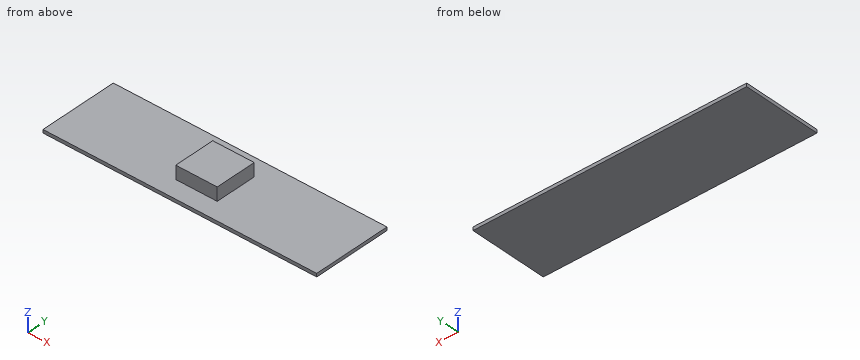
Autodesk Fusion 360 part; units mm, degrees
sketch "Sketch1" plane through (0, 0, 0) normal (0, 0, 1) x (1, 0, 0)
  line L0 (16.5, -4.75) -> (-16.5, -4.75)
  line L1 (-16.5, -4.75) -> (-16.5, 4.75)
  line L2 (-16.5, 4.75) -> (16.5, 4.75)
  line L3 (16.5, 4.75) -> (16.5, -4.75)
  line L4 (16.5, -4.75) -> (-16.5, 4.75) construction
  line L5 (-16.5, -4.75) -> (16.5, 4.75) construction
  line L6 (2.5, -2.5) -> (-2.5, -2.5)
  line L7 (-2.5, -2.5) -> (-2.5, 2.5)
  line L8 (-2.5, 2.5) -> (2.5, 2.5)
  line L9 (2.5, 2.5) -> (2.5, -2.5)
  line L10 (2.5, -2.5) -> (-2.5, 2.5) construction
  line L11 (-2.5, -2.5) -> (2.5, 2.5) construction
  dimension "d1" = 14
  dimension "d2" = 14
  dimension "d3" = 5
  dimension "d4" = 5
  dimension "d5" = 9.5
  dimension "d6" = 33
extrude "Extrude1" add sketch "Sketch1" against normal blind 0.4 contours L0 L1 L2 L3 | L6 L7 L8 L9
extrude "Extrude2" add sketch "Sketch1" along normal blind 1.6 contours L6 L7 L8 L9
Model file for the job. Use its own axes, mm. Give positions to 0.01 mm unless a question says otherwise; leave off trailing zeros. Loops run counter-clockwise (first coordinate to the right, second up) from the corner with the lowest first, then second, coordinate; pieces in that order, holes last. Notation, with made-up numbers: (18, 7.25) -> (60, 7.25) arc R14 ccw to (60, 24.25) -> close; hole circle Ø4 at (36.25, -15.5). An arc over 180 degrees is marked (long way). Use CSV: the item, a comma, the result in double quotes. Start each with the question number.
1) Wall check: line 1 (X direction, y = -0.5, z = 0.15); line 2 (Z direction, x = 13.5, y = -1). Give the ranges that are in metal, low to high.
2) Flat gauge pins, fed straight in: pin 1 Ø5 at (x, y) = (6, -1.5) entering from +Z; pin 2 Ø0.8 at (y, z) = (0.5, 0.5) entering from +X; pin 3 Ø0.8 at (x, z) = (0, 1) entering from -Y. Where does each tip first touch, or does it go through?
3) Slice it at C-C on x = 10. Give the cut face in (y, z).
4) Slice it at B-B on z = 0.6. Give the cut face in (x, y), plus the area to 3 significant figures.
5) Slice it at A-A on y = -1. Give the cut face in (x, z).
Computed values:
1,line 1,"x = -2.5 to 2.5"
1,line 2,"z = -0.4 to 0"
2,pin 1,"stops at z = 0"
2,pin 2,"stops at x = 2.5"
2,pin 3,"stops at y = -2.5"
3,outline,"(-4.75, -0.4) -> (4.75, -0.4) -> (4.75, 0) -> (-4.75, 0) -> close"
4,outline,"(-2.5, -2.5) -> (2.5, -2.5) -> (2.5, 2.5) -> (-2.5, 2.5) -> close"
4,area,"25.0 mm^2"
5,outline,"(-16.5, -0.4) -> (16.5, -0.4) -> (16.5, 0) -> (2.5, 0) -> (2.5, 1.6) -> (-2.5, 1.6) -> (-2.5, 0) -> (-16.5, 0) -> close"
